from build123d import *

# Parameters (mm, degrees)
SKETCH3_W           = 15
SKETCH3_H           = 30
BOSS_EXTRUDE2_DEPTH = 100
CUT_EXTRUDE1_DEPTH  = 104.591746776
BOSS_EXTRUDE3_DEPTH = 5
BOSS_EXTRUDE4_START = 8.5
BOSS_EXTRUDE4_DEPTH = 8.5
FILLET1_R           = 5
SKETCH8_W           = 20
SKETCH8_H           = 13.5
CUT_EXTRUDE3_DEPTH  = 113.722003176
SKETCH10_W          = 5
SKETCH10_H          = 30
BOSS_EXTRUDE5_DEPTH = 35
BOSS_EXTRUDE6_DEPTH = 8.5
SKETCH12_R          = 2.75
CUT_EXTRUDE4_DEPTH  = 119.679189414
FILLET2_R           = 5
BOSS_EXTRUDE7_DEPTH = 5
BOSS_EXTRUDE8_DEPTH = 5


with BuildPart() as part:
    # Sketch3 → Boss-Extrude2 (new body)
    with BuildSketch(Plane.XY):
        with Locations((0, 7.5)):
            Rectangle(SKETCH3_W, SKETCH3_H)
        with BuildLine():
            Line((-3.5, 0), (-3.5, 15))
            ThreePointArc((-3.5, 15), (0, 18.5), (3.5, 15))
            Line((3.5, 15), (3.5, 0))
            ThreePointArc((3.5, 0), (0, -3.5), (-3.5, 0))
        make_face(mode=Mode.SUBTRACT)
    extrude(amount=BOSS_EXTRUDE2_DEPTH)

    # Sketch4 → Cut-Extrude1 (cut, through all)
    with BuildSketch(Plane.ZY.offset(7.5)):
        with BuildLine():
            Line((10, 9.75), (90, 9.75))
            ThreePointArc((90, 9.75), (92.25, 7.5), (90, 5.25))
            Line((90, 5.25), (10, 5.25))
            ThreePointArc((10, 5.25), (7.75, 7.5), (10, 9.75))
        make_face()
    extrude(amount=-CUT_EXTRUDE1_DEPTH, mode=Mode.SUBTRACT)

    # Sketch5 → Boss-Extrude3 (add)
    with BuildSketch(Plane(origin=(0, 0, 0), x_dir=(-1, 0, 0), z_dir=(0, 0, -1))):
        with BuildLine():
            Line((-7.5, -7.5), (-7.5, 7.5))
            Line((-7.5, 7.5), (-7.5, 22.5))
            Line((-7.5, 22.5), (-14, 22.5))
            Line((-14, 22.5), (-37.5, 22.5))
            ThreePointArc((-37.5, 22.5), (-41.035533906, 21.035533906), (-42.5, 17.5))
            Line((-42.5, 17.5), (-42.5, -2.5))
            ThreePointArc((-42.5, -2.5), (-41.035533906, -6.035533906), (-37.5, -7.5))
            Line((-37.5, -7.5), (-14, -7.5))
            Line((-14, -7.5), (-7.5, -7.5))
        make_face()
    extrude(amount=-BOSS_EXTRUDE3_DEPTH)

    # Sketch6 → Boss-Extrude4 (add)
    with BuildSketch(Plane(origin=(0, 0, 0), x_dir=(-1, 0, 0), z_dir=(0, 0, -1)).offset(BOSS_EXTRUDE4_START)):
        with BuildLine():
            Line((-8.122776602, 22.5), (-37.5, 22.5))
            ThreePointArc((-37.5, 22.5), (-41.035533906, 21.035533906), (-42.5, 17.5))
            Line((-42.5, 17.5), (-42.5, -2.5))
            ThreePointArc((-42.5, -2.5), (-41.035533906, -6.035533906), (-37.5, -7.5))
            Line((-37.5, -7.5), (-8.122776602, -7.5))
            ThreePointArc((-8.122776602, -7.5), (-11.5, 7.5), (-8.122776602, 22.5))
        make_face()
    extrude(amount=-BOSS_EXTRUDE4_DEPTH)

    # Fillet1
    fillet1_edges = [part.edges().sort_by_distance(p)[0] for p in [
        (8.122776602, -7.5, -4.25),
        (8.122776602, 22.5, -4.25),
    ]]
    fillet(fillet1_edges, radius=FILLET1_R)

    # Sketch8 → Cut-Extrude3 (cut, through all)
    with BuildSketch(Plane(origin=(0, 22.5, 0), x_dir=(1, 0, 0), z_dir=(0, 1, 0))):
        with Locations((17.5, 1.75)):
            Rectangle(SKETCH8_W, SKETCH8_H)
    extrude(amount=-CUT_EXTRUDE3_DEPTH, mode=Mode.SUBTRACT)


with BuildPart() as cut_extrude3_piece_1:
    # of the separate pieces the step leaves, piece 1, a body of its own (cut_extrude3_pieces)
    add(part.part.solids().sort_by_distance((-7.5, -7.5, 100))[0])

    # Sketch10 → Boss-Extrude5 (add)
    with BuildSketch(Plane(origin=(7.5, 0, 0), x_dir=(0, 0, -1), z_dir=(1, 0, 0))):
        with Locations((-2.5, 7.5)):
            Rectangle(SKETCH10_W, SKETCH10_H)
    extrude(amount=BOSS_EXTRUDE5_DEPTH)

    # Sketch11 → Boss-Extrude6 (add)
    with BuildSketch(Plane(origin=(0, 0, 0), x_dir=(-1, 0, 0), z_dir=(0, 0, -1))):
        with BuildLine():
            Line((-42.5, -7.5), (-22.5, -7.5))
            Line((-22.5, -7.5), (-19.314112746, -7.5))
            ThreePointArc((-19.314112746, -7.5), (-21.865716684, 7.5), (-19.314112746, 22.5))
            Line((-19.314112746, 22.5), (-22.5, 22.5))
            Line((-22.5, 22.5), (-42.5, 22.5))
            Line((-42.5, 22.5), (-42.5, -7.5))
        make_face()
    extrude(amount=BOSS_EXTRUDE6_DEPTH)

    # Sketch12 → Cut-Extrude4 (cut, through all)
    with BuildSketch(Plane(origin=(0, 0, -8.5), x_dir=(-1, 0, 0), z_dir=(0, 0, -1))):
        with Locations((-29.682858342, 0)):
            Circle(SKETCH12_R)
        with Locations((-29.682858342, 15)):
            Circle(SKETCH12_R)
    extrude(amount=-CUT_EXTRUDE4_DEPTH, mode=Mode.SUBTRACT)

    # Fillet2
    fillet2_edges = [cut_extrude3_piece_1.edges().sort_by_distance(p)[0] for p in [
        (42.5, -7.5, -1.75),
        (42.5, 22.5, -1.75),
    ]]
    fillet(fillet2_edges, radius=FILLET2_R)

    # Sketch13 → Boss-Extrude7 (add)
    with BuildSketch(Plane.XZ.offset(7.5)):
        Polygon((7.5, 5), (7.5, 20), (22.5, 5), align=None)
    extrude(amount=-BOSS_EXTRUDE7_DEPTH)

    # Sketch14 → Boss-Extrude8 (add)
    with BuildSketch(Plane(origin=(0, 22.5, 0), x_dir=(1, 0, 0), z_dir=(0, 1, 0))):
        Polygon((22.5, -5), (7.5, -5), (7.5, -20), align=None)
    extrude(amount=-BOSS_EXTRUDE8_DEPTH)


with BuildPart() as cut_extrude3_piece_2:
    # of the separate pieces the step leaves, piece 2, a body of its own (cut_extrude3_pieces)
    add(part.part.solids().sort_by_distance((37.5, -7.5, -8.5))[0])


solid = cut_extrude3_piece_1.part
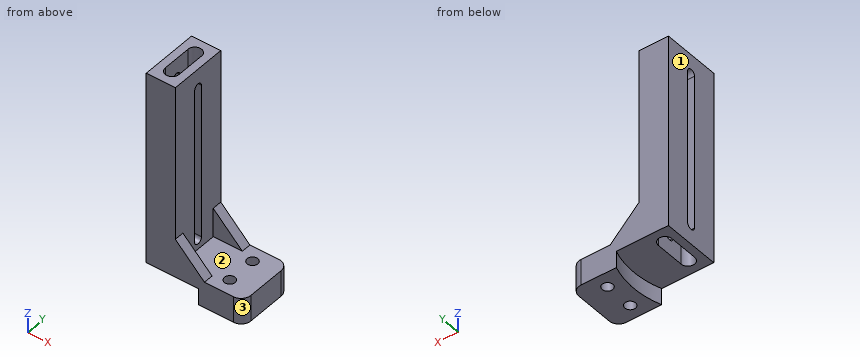
The listing builds one solid part. Answer for the finished solid, in the listing's coordinates (mm). Face numbers are marked on the shaded views. Coordinates: 2 decimals unless noted, no trailing zeros. Loops run counter-clockwise (first coordinate to the right, second up) from the corner with the lowest first, then second, coordinate; pieces in that order, holes last. Notation, with made-up numbers: (8.25, 40.25) -> (47.25, 40.25) arc R21 cw to (47.25, 76.25) -> close; hole circle Ø10 at (28.25, 80). An arc over 180 degrees is marked (long way). Write item = value, one per line. Start each with the question number.
1) Straight lines are drawn through the part: line 1 (Y direction, x = -5, z = 34); line 2 (X direction, y = 8.75, z = 93); line 3 (Y direction, x = 14, z = 13). For each, find the intervals that lie inside material, in ascending order. Write a range as from..to.
2) A cutting plane is placed at A-A (z = 48.5). Give the vertices of the cut face in (x, y), then the cut area to 3 significant figures.
3) A cutting plane is placed at D-D (y = 20). Give the vertices of the cut face in (x, z), then the cut area to 3 significant figures.
4) A cutting plane is placed at C-C (x = 11.5). Give the vertices of the cut face in (y, z).
5) Given pin 1 Ø12 at (x, y) = (16.5, 16) entering from +Z; pin 2 Ø7 at (x, y) = (29.68, 0) entering from +Z; pin 3 Ø9 at (y, z) = (1.5, 69.5) entering from +X, each flat-ended and moving along its own axis, determine where each tip first touches the part or whether it passes through.
6) The mould has two halves that part along Y. Classify the marked faces 1, 2 and 3: released by +Y, released by -Y, zero draft, split by the parting line, or undercut.
7) A cutting plane is placed at B-B (y = 7.5). Give the vertices of the cut face in (x, z), then the cut area to 3 significant figures.
Responses:
q1.line_1 = -7.5..5.25, 9.75..22.5
q1.line_2 = -7.5..-3.5, 3.5..7.5
q1.line_3 = -7.5..-2.5, 17.5..22.5
q2.outline = (-7.5, -7.5) -> (7.5, -7.5) -> (7.5, 5.25) -> (3.5, 5.25) -> (3.5, 0) arc R3.5 cw to (-3.5, 0) -> (-3.5, 5.25) -> (-7.5, 5.25) -> close; (-7.5, 9.75) -> (-3.5, 9.75) -> (-3.5, 15) arc R3.5 cw to (3.5, 15) -> (3.5, 9.75) -> (7.5, 9.75) -> (7.5, 22.5) -> (-7.5, 22.5) -> close
q2.area = 271 mm²
q3.outline = (-7.5, 0) -> (20.11, 0) -> (20.11, -8.5) -> (41.83, -8.5) -> (41.83, 5) -> (22.5, 5) -> (7.5, 20) -> (7.5, 100) -> (-7.5, 100) -> close
q3.area = 1,970 mm²
q4.outline = (-7.5, 0) -> (22.5, 0) -> (22.5, 16) -> (17.5, 16) -> (17.5, 5) -> (-2.5, 5) -> (-2.5, 16) -> (-7.5, 16) -> close
q5.pin_1 = 16.81
q5.pin_2 = 5
q5.pin_3 = 7.5
q6.face_1 = zero draft
q6.face_2 = undercut
q6.face_3 = released by -Y
q7.outline = (-7.5, 0) -> (-3.5, 0) -> (-3.5, 7.75) -> (-7.5, 7.75) -> close; (-7.5, 92.25) -> (-3.5, 92.25) -> (-3.5, 100) -> (-7.5, 100) -> close; (3.5, 0) -> (21.87, 0) -> (21.87, -8.5) -> (42.5, -8.5) -> (42.5, 5) -> (7.5, 5) -> (7.5, 7.75) -> (3.5, 7.75) -> close; (3.5, 92.25) -> (7.5, 92.25) -> (7.5, 100) -> (3.5, 100) -> close
q7.area = 474 mm²
